Print and shaded views of the part. All mm, measured from the part's lowest x, y and z. Round coordinates to 2 decimals unless told otherwise and drop trailing zeros. Write each loop counter-clockwise with the first axis right and the second up, starting at its lowest first coordinate (ties: lowest second). Pieces come first, ordered by that corner, then holes. Notation, with made-up numbers: M 55.25,29.5 L 79.25,29.5 A22 ccw 79.25,45.5 Z; hole C 18.25,10.25 d6. An arc over 180 degrees is marked long. Write item = value, one per line. Start each with the question number.
Q1. Band-saw the part on C-C on x = 12.7. Write the cut outline in (y, z) (3 decimals).
Q2. Drop flat-ended pins along their axis: P1, Ø5, axis at x = 22.5, y = 18.5, coming from the -Z side; P2, Ø3, axis at x = 13, y = 9.5, coming from the +Z side. Give the stop position or say it passes through.
Q3. Band-saw the part on B-B on y = 7.62. Write the cut outline in (x, z).
Q4. Band-saw the part on D-D on x = 7. Write the cut outline in (y, z), plus the area to 3 significant figures.
Q5. Pull direction X, two halves, no side cores. Call the marked faces 1, 2 and 3: released by +X, released by -X, zero draft, split by the parting line, or undercut.
Q6. Band-saw the part on A-A on z = 7.62. Write the cut outline in (x, y) (3 decimals), plus the area to 3 significant figures.
Q7. Probe L1, parallel to Y at x = 5.75, z = 7.62; L2, parallel to X at y = 25, z = 7.5; L3, parallel to Y at x = 24, z = 2.5. List the from-to ranges inside material, lowest first.
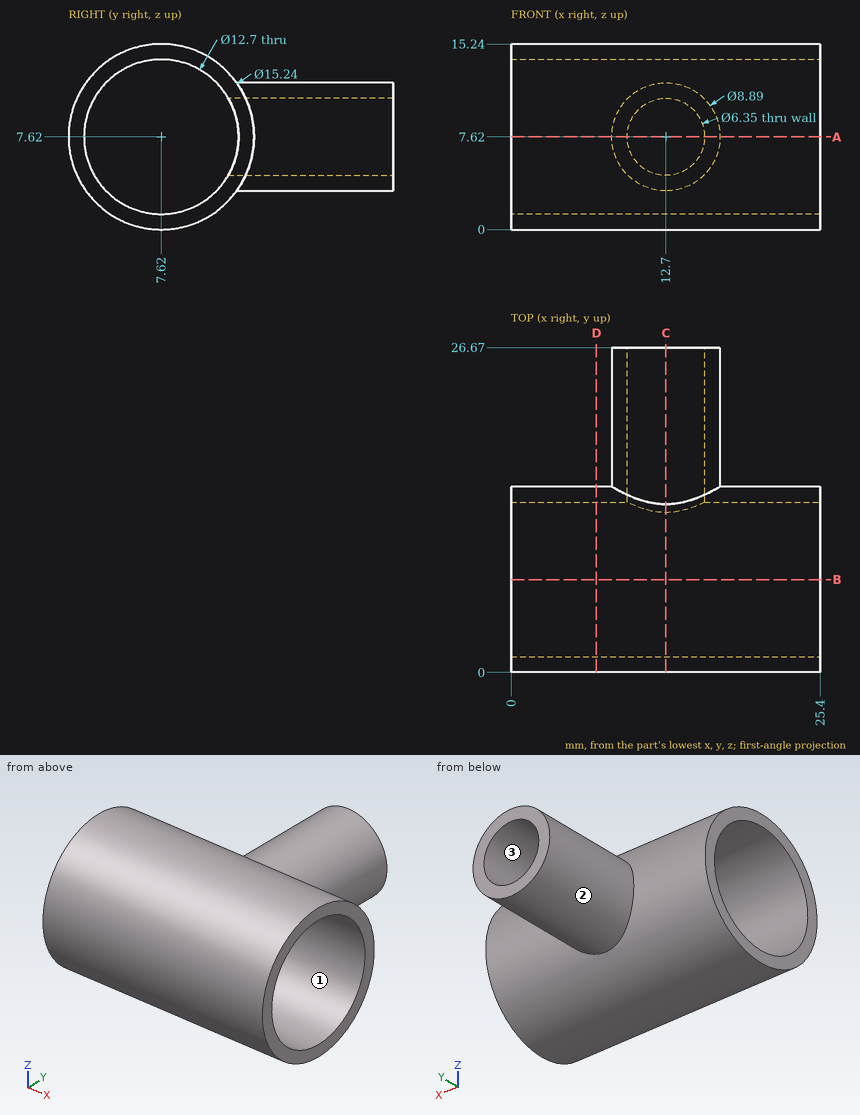
Conclusion:
q1.outline = M 13.119,4.445 A6.35 cw long 13.119,10.795 L 26.67,10.795 L 26.67,12.065 L 13.809,12.065 A7.62 ccw long 13.809,3.175 L 26.67,3.175 L 26.67,4.445 Z
q2.P1 = through
q2.P2 = 15.23
q3.outline = M 0,0 L 25.4,0 L 25.4,1.27 L 0,1.27 Z; M 0,13.97 L 25.4,13.97 L 25.4,15.24 L 0,15.24 Z
q4.outline = C 7.62,7.62 d15.24; hole C 7.62,7.62 d12.7
q4.area = 55.7 mm^2
q5.face_1 = zero draft
q5.face_2 = split by the parting line
q5.face_3 = undercut
q6.outline = M 0,0 L 25.4,0 L 25.4,1.27 L 0,1.27 Z; M 0,13.97 L 9.525,13.97 L 9.525,26.67 L 8.255,26.67 L 8.255,15.24 L 0,15.24 Z; M 15.875,13.97 L 25.4,13.97 L 25.4,15.24 L 17.145,15.24 L 17.145,26.67 L 15.875,26.67 Z
q6.area = 85.5 mm^2
q7.L1 = 0 to 1.27, 13.97 to 15.24
q7.L2 = 8.26 to 9.53, 15.87 to 17.14
q7.L3 = 1.98 to 3.86, 11.38 to 13.26
